Part model, mm, in its own coordinate system. Face numbers are marked on the shaded views. A direction names the side the tool comes from. Round coordinates to 2 decimals unless told otherwise and drop trailing zeros. Write each loop counter-clockwise with the first axis right and the second up, starting at its lowest first coordinate (ties: lowest second). Pieces come first, ordered by that corner, then holes.
1) Saw through at D-D on z = -5. Write the cut outline in (x, y), and give its area (3 significant figures).
2) Pull direction X, two halves, no side cores. Call the marked faces 1, 2, 3 and 4: +X half, -X half, draft (parallel to the pull), parting line (faces both ways), or undercut.
3) Which spindle directions (+Z, -Z, +X, -X, +Y, -Y) get a long thin tool onto all of the face, cutting with end or side? Do the marked faces 5, 6 and 7. Say none if no direction does.
4) Drill centre lines: L1, parallel to X at y = 22, z = 0; L2, parallel to Y at x = 0, z = -8.75; L3, parallel to Z at x = 1.55, y = 26.5. Where is each one in solid material? Low to high.
5) Saw through at B-B on y = 15. Write the cut outline in (x, z).
6) Saw through at C-C on z = 0. Write the cut outline in (x, y).
7) Saw through at A-A on x = 0. Write the cut outline in (y, z), and give its area (3 significant figures).
8) Flat gauge pins, fed straight in: pin 1 (4 mm diameter, centred on y = 9.5, z = -7.5, fed in from -X); pin 2 (1.4 mm diameter, centred on x = -0.5, y = 15, fed in from -Z); pin 3 (1.8 mm diameter, centred on x = 0, z = -10, fed in from -Y). Where does each tip first touch, or does it go through?
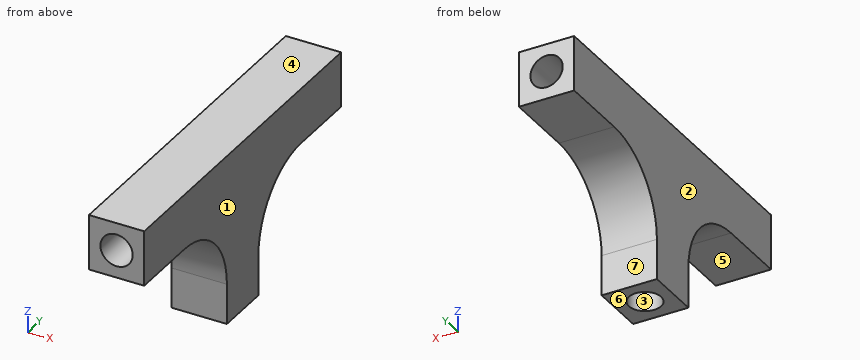
Autodesk Fusion 360 part; units mm, degrees
sketch "スケッチ2" plane through (0, 0, 0) normal (0, 1, 0) x (1, 0, 0)
  circle A0 centre (0, 0) radius 1.4
  circle A1 centre (0, 0) radius 2.4
  line L0 (2.4, -2.4) -> (-2.4, -2.4)
  line L1 (-2.4, -2.4) -> (-2.4, 2.4)
  line L2 (-2.4, 2.4) -> (2.4, 2.4)
  line L3 (2.4, 2.4) -> (2.4, -2.4)
  dimension "d1" = 2.8
  dimension "d2" = 1
extrude "押し出し1" add sketch "スケッチ2" along normal blind 30
sketch "スケッチ3" plane through (0, 0, -2.4) normal (0, 0, -1) x (-1, 0, 0)
  circle A0 centre (0, 15) radius 1.4
  circle A1 centre (0, 15) radius 2.4
  line L0 (0, 30) -> (0, 0) construction
  line L1 (2.25, 30) -> (-2.25, 30) construction
  line L2 (-2.4, 0) -> (2.4, 0)
  line L3 (2.4, 0) -> (2.4, 30)
  line L4 (2.4, 30) -> (-2.4, 30)
  line L5 (-2.4, 30) -> (-2.4, 0)
  line L6 (2.4, 12.6) -> (-2.4, 12.6)
  line L7 (-2.4, 12.6) -> (-2.4, 17.4)
  line L8 (-2.4, 17.4) -> (2.4, 17.4)
  line L9 (2.4, 17.4) -> (2.4, 12.6)
  dimension "d6" = 2.8
  dimension "d7" = 1
extrude "押し出し2" add sketch "スケッチ3" along normal blind 10 contours A1 | A1 L3 L6 L9 | A1 L3 L8 L9 | A1 L5 L7 L8 | A1 L5 L6 L7
fillet "フィレット1" radius 6.5 1 edges at (0, 12.6, -2.4)
fillet "フィレット2" radius 6.5 1 edges at (0, 17.4, -2.4)
Completed:
1. outline: (-2.4, 11.3) - (2.4, 11.3) - (2.4, 18.7) - (-2.4, 18.7) - close; hole circle Ø2.8 at (0, 15)
1. area: 29.4 mm2
2. face 1: +X half
2. face 2: -X half
2. face 3: undercut
2. face 4: draft
3. face 5: -Z, +X, -X, -Y
3. face 6: -Z, +X, -X, +Y, -Y
3. face 7: -Z, +X, -X, +Y
4. L1: x = -2.4 to -1.4, 1.4 to 2.4
4. L2: y = 12.6 to 13.6, 16.4 to 17.4
4. L3: z = -2.4 to 2.4
5. outline: (-2.4, -12.4) - (-1.4, -12.4) - (-1.4, -2.4) - (1.4, -2.4) - (1.4, -12.4) - (2.4, -12.4) - (2.4, 2.4) - (-2.4, 2.4) - close; hole circle Ø2.8 at (0, 0)
6. outline: (-2.4, 0) - (-1.4, 0) - (-1.4, 30) - (-2.4, 30) - close; (1.4, 0) - (2.4, 0) - (2.4, 30) - (1.4, 30) - close
7. outline: (0, -2.4) - (6.1, -2.4) arc R6.5 cw to (12.6, -8.9) - (12.6, -12.4) - (13.6, -12.4) - (13.6, -2.4) - (16.4, -2.4) - (16.4, -12.4) - (17.4, -12.4) - (17.4, -8.9) arc R6.5 cw to (23.9, -2.4) - (30, -2.4) - (30, -1.4) - (0, -1.4) - close; (0, 1.4) - (30, 1.4) - (30, 2.4) - (0, 2.4) - close
7. area: 98.1 mm2
8. pin 1: passes through
8. pin 2: stops at z = -2.4
8. pin 3: stops at y = 12.6
